```python
from build123d import *

# Parameters (mm, degrees)
F1_DEPTH = 3
F3_DEPTH = 21
F4_R     = 1.5
F5_DEPTH = 4
F7_DEPTH = 5


with BuildPart() as f1:
    # F0 (on Top) → F1 (new body)
    with BuildSketch(Plane.XY):
        with BuildLine():
            Line((12.5, 54.75), (12.5, 73.697439))
            ThreePointArc((12.5, 73.697439), (0, 74.75), (-12.5, 73.697439))
            Line((-12.5, 73.697439), (-12.5, 54.75))
            Line((-12.5, 54.75), (8.383245, 54.75))
            Line((8.383245, 54.75), (12.5, 54.75))
        make_face()
    extrude(amount=F1_DEPTH)

    # F2 (on face) → F3 (join)
    with BuildSketch(Plane.XY.offset(3)):
        with BuildLine():
            Line((-12.5, 73.697439), (-12.5, 54.75))
            Line((-12.5, 54.75), (-8.5, 54.75))
            Line((-8.5, 54.75), (-8.5, 71.25))
            Line((-8.5, 71.25), (8.5, 71.25))
            Line((8.5, 71.25), (8.5, 54.75))
            Line((8.5, 54.75), (12.5, 54.75))
            Line((12.5, 54.75), (12.5, 73.697439))
            ThreePointArc((12.5, 73.697439), (0, 74.75), (-12.5, 73.697439))
        make_face()
    extrude(amount=F3_DEPTH)

    # F4 (on face) → F5 (cut)
    with BuildSketch(Plane.XY.offset(3)):
        with BuildLine():
            ThreePointArc((6.5, 64.75), (5, 66.25), (3.5, 64.75))
            ThreePointArc((3.5, 64.75), (5, 63.25), (6.5, 64.75))
        make_face()
        with Locations((-5, 64.75)):
            Circle(F4_R)
    extrude(amount=-F5_DEPTH, mode=Mode.SUBTRACT)

    # F6 (on face) → F7 (cut)
    with BuildSketch(Plane.XZ.offset(-71.25)):
        with BuildLine():
            ThreePointArc((1.5, 13), (1.06066, 14.06066), (0, 14.5))
            ThreePointArc((0, 14.5), (-1.06066, 11.93934), (1.5, 13))
        make_face()
    extrude(amount=-F7_DEPTH, mode=Mode.SUBTRACT)


solid = f1.part
```
For this review, take the finished solid that the model builds, in its own axes (mm). A direction names the side the tool comes from. Coordinates: 2 decimals unless noted, no trailing zeros. Loops run counter-clockwise (first coordinate to the right, second up) from the corner with the lowest first, then second, coordinate; pieces in that order, holes last.
1. Add section A-A, the plane y = 64.75. Give the boundary of the cut face in (x, z).
2. Insertion check: P1, Ø1.5, axis at x = 1, z = 12.5, coming from the +Y side; P2, Ø5, axis at x = 0, z = 13, coming from the +Y side; P3, Ø1.5, axis at x = -3, y = 66, coming from the +Z side. Each pin has a flat end and moves straight along its axis. Give the tip position at first contact, or say it passes through.
3. Add section C-C, the plane x = 0.75. Give the boundary of the cut face in (y, z).
4. For line 1 (X direction, y = 64.75, z = 1.6); line 2 (X direction, y = 63.75, z = 2); line 3 (X direction, y = 56.75, z = 13), list the stretches that pass through material, from the lowest coordinate up.
5. Add section D-D, the plane y = 56. Give the boundary of the cut face in (x, z), then the cut area to 3 significant figures.
6. For faces 1 (the flat face through (-12.5, 64, 12)), 2 (the flat face through (-2, 71.25, 13)), list the 3-axis set-ups (+Z, -Z, +X, -X, +Y, -Y) from which the entire face can be reached by the end or side of a thin tool; tool diameter is ignored.
7. Add section B-B, the plane z = 18.5. Give the boundary of the cut face in (x, y), then the cut area to 3 significant figures.
8. Mouldability with a two-part tool opening along Y and no side actions: class faces 3 (the flat face through (8.5, 63, 13)), 4 (the cylindrical face through (5.195, 63.263, 1.521)), 5 (the flat face through (-9, 54.75, 9)) as +Y half, -Y half, draft (parallel to the pull), parting line (faces both ways), or undercut.
Result:
1. outline: (-12.5, 0) - (-6.5, 0) - (-6.5, 3) - (-8.5, 3) - (-8.5, 24) - (-12.5, 24) - close; (-3.5, 0) - (3.5, 0) - (3.5, 3) - (-3.5, 3) - close; (6.5, 0) - (12.5, 0) - (12.5, 24) - (8.5, 24) - (8.5, 3) - (6.5, 3) - close
2. P1: stops at y = 74.75
2. P2: stops at y = 74.75
2. P3: stops at z = 3
3. outline: (54.75, 0) - (74.75, 0) - (74.75, 11.7) - (71.25, 11.7) - (71.25, 3) - (54.75, 3) - close; (71.25, 14.3) - (74.75, 14.3) - (74.75, 24) - (71.25, 24) - close
4. line 1: x = -12.5 to -6.5, -3.5 to 3.5, 6.5 to 12.5
4. line 2: x = -12.5 to -6.12, -3.88 to 3.88, 6.12 to 12.5
4. line 3: x = -12.5 to -8.5, 8.5 to 12.5
5. outline: (-12.5, 0) - (12.5, 0) - (12.5, 24) - (8.5, 24) - (8.5, 3) - (-8.5, 3) - (-8.5, 24) - (-12.5, 24) - close
5. area: 243 mm2
6. face 1: +Z, -Z, -X, +Y, -Y
6. face 2: +Z, -Y
7. outline: (-12.5, 54.75) - (-8.5, 54.75) - (-8.5, 71.25) - (8.5, 71.25) - (8.5, 54.75) - (12.5, 54.75) - (12.5, 73.7) arc R74.75 ccw to (-12.5, 73.7) - close
7. area: 211 mm2
8. face 3: draft
8. face 4: undercut
8. face 5: -Y half
